Input: part model. Units: mm. Frame: model coordinates. Coordinates: 2 decimals unless noted, no trailing zeros. Order: outer loops, then holes, each group sorted by start corner. A loop starts at its lowest first (then second) coordinate and runs counter-clockwise, first axis right, second up. Notation, with made-up numbers: M 82.5,65 L 138.5,65 A11 ccw 138.5,70 Z; hole C 75,5 d1. An arc over 180 degrees is marked long. Answer in a Markdown table with one row per item.
Autodesk Fusion 360 part; units mm, degrees
sketch "Sketch1" plane through (0, 0, 0) normal (0, 1, 0) x (1, 0, 0)
  line L0 (-50, 25) -> (10, 25)
  line L1 (10, 25) -> (10, -35)
  line L2 (10, -35) -> (-50, -35)
  line L3 (-50, -35) -> (-50, 25)
  line L4 (-20, -50) -> (-20, 45) construction
  line L5 (30, -5) -> (-85, -5) construction
  line L6 (-85, 17.5) -> (30, 17.5) construction
  line L7 (-85, -27.5) -> (30, -27.5) construction
  circle A0 centre (-40, 17.5) radius 2.55
  circle A1 centre (0, 17.5) radius 2.55
  circle A2 centre (-20, -27.5) radius 2.55
  dimension "d1" = 60
  dimension "d2" = 60
  dimension "d3" = 22.5
  dimension "d4" = 5.1
  dimension "d5" = 5.1
extrude "Extrude1" add sketch "Sketch1" along normal blind 6
sketch "Sketch3" plane through (0, 6, 0) normal (0, 1, 0) x (-1, 0, 0)
  circle A0 centre (40, -17.5) radius 2.55
  circle A1 centre (20, 27.5) radius 2.55
  circle A2 centre (0, -17.5) radius 2.55
  line L0 (50, 35) -> (-10, 35)
  line L1 (-10, 35) -> (-10, -25)
  line L2 (-10, -25) -> (50, -25)
  line L3 (50, -25) -> (50, 35)
equation "d3 = separation / 2"
equation "d4 = hole_01"
equation "d5 = hole_01"
equation "separation = 45 mm"
equation "hole_01 = 5.1 mm"
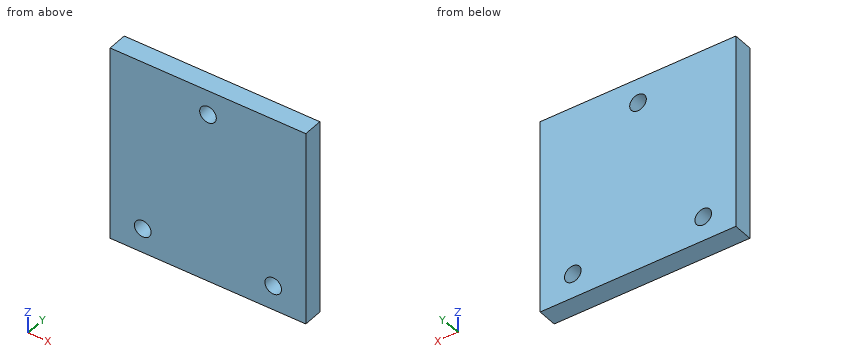
1) Cut plane A-A, the plane x = -40. Output: boundary loops of the cut face in (y, z).
Resolved:
| item | result |
|---|---|
| outline | M 0,-25 L 6,-25 L 6,-20.05 L 0,-20.05 Z; M 0,-14.95 L 6,-14.95 L 6,35 L 0,35 Z |
2) Cut plane C-C, the plane y = 3.3. Output: boundary loops of the cut face in (x, z).
Resolved:
| item | result |
|---|---|
| outline | M -50,-25 L 10,-25 L 10,35 L -50,35 Z; hole C -40,-17.5 d5.1; hole C -20,27.5 d5.1; hole C 0,-17.5 d5.1 |
3) Contact query for a flat-ended pin moving along its axis: pin 1 (4.5 mm diameter, centred on x = 0, z = -17.5, fed in from +Y). Output: stop coordinate, or through.
Resolved:
| item | result |
|---|---|
| pin 1 | passes through |
4) Cut plane B-B, the plane z = 27.5. Output: boundary loops of the cut face in (x, y), and give its area (3 significant figures).
Resolved:
| item | result |
|---|---|
| outline | M -50,0 L -22.55,0 L -22.55,6 L -50,6 Z; M -17.45,0 L 10,0 L 10,6 L -17.45,6 Z |
| area | 329 mm2 |
5) Material intervals for probe 1 along X at (y, z) = (3.5, -17.5); probe 2 along Z at (x, y) = (-40, 2.8); probe 3 along Z at (x, y) = (-20, 4.05), sorted ascending.
Resolved:
| item | result |
|---|---|
| probe 1 | x = -50 to -42.55, -37.45 to -2.55, 2.55 to 10 |
| probe 2 | z = -25 to -20.05, -14.95 to 35 |
| probe 3 | z = -25 to 24.95, 30.05 to 35 |
